Verification items for the finished model (mm, model axes). A direction names the side the tool comes from. Coordinates: 2 decimals unless noted, no trailing zeros. Loops run counter-clockwise (first coordinate to the right, second up) from the corner with the lowest first, then second, coordinate; pieces in that order, holes last.
Q1. Sectioned sample at B-B (z = 28). Enter the section's corners in (x, y), then the cut area to 3 significant figures.
Q2. Access from +Z, -Z, +X, -X, +Y, -Y to the whole of each face (thin tool, end or side, straight path). Record for faces 1 (the face through (-79, 0, 69.7)), 2 (the face through (-79, -9.525, 71)), 3 (the face through (-53.34, 0, 57)).
Q3. Sectioned sample at A-A (y = -11). Enter the section's corners in (x, z), then the cut area to 3 significant figures.
Q4. Sectioned sample at C-C (x = -47). Enter the section's corners in (y, z).
Q5. Material ranges on probe 1 along Z at (x, y) = (3, 5); probe 2 along Z at (x, y) = (-10, 0.75); probe 3 along X at (y, z) = (-8, 72), recorded low to high.
Q6. Go/stop test with flat-tipped pins: P1, Ø6, axis at x = -41, y = -4, coming from the +Z side; P2, Ø6, axis at y = 5, z = 43, coming from the +X side; P3, Ø4, axis at x = -11, y = 4, coming from the +Z side. Record where each tip stops, or that it passes through.
```python
from build123d import *

# Parameters (mm, degrees)
F1_DEPTH = 12.7
F2_W     = 19.05
F2_H     = 3
F3_DEPTH = 6.35
F4_W     = 19.05
F4_H     = 3
F5_DEPTH = 6.35
F6_SIZE  = 0.5


with BuildPart() as f1:
    # F0 (on Front) → F1 (new body, symmetric)
    with BuildSketch(Plane.XZ):
        Polygon((0, -10), (0, 0), (0, 7.62), (-7.62, 7.62), (-7.62, 15.24), (-15.24, 15.24), (-15.24, 22.86), (-22.86, 22.86), (-22.86, 30.48), (-30.48, 30.48), (-30.48, 38.1), (-38.1, 38.1), (-38.1, 45.72), (-45.72, 45.72), (-45.72, 53.34), (-53.34, 53.34), (-53.34, 60.96), (-60.96, 60.96), (-60.96, 68.58), (-68.58, 68.58), (-68.58, 76.2), (-76.2, 76.2), (-76.2, 66.2), align=None)
    extrude(amount=F1_DEPTH, both=True)

    # F2 (on face) → F3 (join)
    with BuildSketch(Plane.YZ):
        with Locations((0, -5)):
            Rectangle(F2_W, F2_H)
    extrude(amount=F3_DEPTH)

    # F4 (on face) → F5 (join)
    with BuildSketch(Plane(origin=(-76.2, 0, 0), x_dir=(0, -1, 0), z_dir=(-1, 0, 0))):
        with Locations((0, 71.2)):
            Rectangle(F4_W, F4_H)
    extrude(amount=F5_DEPTH)

    # F6
    f6_edges = [f1.edges().sort_by_distance(p)[0] for p in [
        (-82.55, 0, 72.7),
        (-82.55, 9.525, 71.2),
        (-82.55, 0, 69.7),
        (-82.55, -9.525, 71.2),
        (6.35, 9.525, -5),
        (6.35, 0, -3.5),
        (6.35, -9.525, -5),
        (6.35, 0, -6.5),
    ]]
    chamfer(f6_edges, length=F6_SIZE)


solid = f1.part
```
Geometry check:
1. outline: (-38, -12.7) - (-22.86, -12.7) - (-22.86, 12.7) - (-38, 12.7) - close
1. area: 385 mm2
2. face 1: -Z, -X, +Y, -Y
2. face 2: +Z, -Z, -X, -Y
2. face 3: +Z, +X, +Y, -Y
3. outline: (-76.2, 66.2) - (0, -10) - (0, 7.62) - (-7.62, 7.62) - (-7.62, 15.24) - (-15.24, 15.24) - (-15.24, 22.86) - (-22.86, 22.86) - (-22.86, 30.48) - (-30.48, 30.48) - (-30.48, 38.1) - (-38.1, 38.1) - (-38.1, 45.72) - (-45.72, 45.72) - (-45.72, 53.34) - (-53.34, 53.34) - (-53.34, 60.96) - (-60.96, 60.96) - (-60.96, 68.58) - (-68.58, 68.58) - (-68.58, 76.2) - (-76.2, 76.2) - close
3. area: 1,050 mm2
4. outline: (-12.7, 37) - (12.7, 37) - (12.7, 53.34) - (-12.7, 53.34) - close
5. probe 1: z = -6.5 to -3.5
5. probe 2: z = 0 to 15.24
5. probe 3: x = -82.55 to -68.58
6. P1: stops at z = 45.72
6. P2: stops at x = -38.1
6. P3: stops at z = 15.24
